Read the model definition and answer for the solid it produces. Units are mm, in the model's axes. Face numbers are marked on the shaded views. A direction names the side the tool comes from. Round coordinates to 2 decimals unless told otherwise and drop trailing zeros. Write each loop counter-clockwise with the first axis right and the second up, starting at its lowest first coordinate (ties: lowest second). Pieces come first, ordered by that corner, then holes. Notation, with made-up numbers: (61.5, 86) - (114.5, 86) arc R25 cw to (114.5, 119) - close; hole circle Ø8 at (73.5, -33.5). An arc over 180 degrees is marked (long way). Answer as CSV lines item,"result". Start each with the question number.
1) Which of the six approach directions +Z, -Z, +X, -X, +Y, -Y give full straight-line access (tool end or side, diameter ignored) to the marked faces 5 and 6?
2) Find section D-D on x = 16.5. Determine the outline of the cut face in (y, z), then the cut area to 3 significant figures.
3) Consider line 1 along Z through (x, y) = (-17, 6.5); line 2 along Y through (x, z) = (-32.5, 33.5); line 3 along Z through (x, y) = (-34, 47.5). Determine where each line is inside the solid, lowest interval first.
4) Find section B-B on x = 31. Determine the outline of the cut face in (y, z), then the cut area to 3 significant figures.
5) For a pull along X with two mould halves and no side action, classify the marked faces 1, 2, 3 and 4 as +X half, -X half, draft (parallel to the pull), parting line (faces both ways), or undercut.
6) Find section A-A on z = 4.5. Determine the outline of the cut face in (x, y), then the cut area to 3 significant figures.
7) Each of these flat-tipped pins is pushed along its axis until it touches: pin 1 (4.5 mm diameter, centred on x = -36, y = -2.5, fed in from -Z); pin 2 (1.2 mm diameter, centred on x = -14.5, z = 26, fed in from -Y); pin 3 (23 mm diameter, centred on x = 3.5, y = 30, fed in from +Z). Where does it stop, or does it pass through?
8) Find section C-C on y = -3. Determine the outline of the cut face in (x, z), then the cut area to 3 significant figures.
from build123d import *

# Parameters (mm, degrees)
F0_W      = 76.35137
F0_H      = 104.6798825264
F1_DEPTH  = 20
F3_DEPTH  = 105
F4_W      = 93.6356825264
F4_H      = 10
F5_DEPTH  = 100
F7_DEPTH  = 25
F6_W      = 71.0693526958
F6_H      = 99.8780601819
F8_DEPTH  = 5
F9_W      = 29.2911557481
F9_H      = 16.3262225688
F9_W_2    = 29.291
F10_DEPTH = 4
F11_R     = 1.65


with BuildPart() as f1:
    # F0 (on Top) → F1 (new body)
    with BuildSketch(Plane.XY):
        with Locations((-0.238945, 18.4870436788)):
            Rectangle(F0_W, F0_H)
    extrude(amount=F1_DEPTH)

    # F2 (on face) → F3 (cut)
    with BuildSketch(Plane.XZ.offset(33.8528975844)):
        Polygon((32.4146378825, 10.8041167259), (-32.89253, 10.8041167259), (-32.89253, 9.3744061509), (-32.89253, 0), (32.4146378825, 0), (32.4146378825, 9.3744061509), align=None)
    extrude(amount=-F3_DEPTH, mode=Mode.SUBTRACT)

    # F4 (on face) → F5 (cut)
    with BuildSketch(Plane(origin=(-38.41463, 0, 0), x_dir=(0, -1, 0), z_dir=(-1, 0, 0))):
        with Locations((-18.4870436788, 5)):
            Rectangle(F4_W, F4_H)
    extrude(amount=-F5_DEPTH, mode=Mode.SUBTRACT)

    # F6 (on face) → F7 (join)
    with BuildSketch(Plane.XY.offset(20)):
        Polygon((-38.41463, 68.4260725975), (-35.7736226958, 68.4260725975), (35.29573, 68.4260725975), (37.93674, 68.4260725975), (37.93674, 70.826984942), (-38.41463, 70.826984942), align=None)
    extrude(amount=F7_DEPTH)

    # F6 (on face) → F8 (join)
    with BuildSketch(Plane.XY.offset(20)):
        with Locations((-0.2389463479, 18.4870425065)):
            Rectangle(F6_W, F6_H)
    extrude(amount=F8_DEPTH)

    # F9 (on face) → F10 (join)
    with BuildSketch(Plane.XY.offset(25)):
        with Locations((-17.5266725798, 57.14177154)):
            Rectangle(F9_W, F9_H)
        with Locations((14.4065536521, 57.14177154)):
            Rectangle(F9_W_2, F9_H)
    extrude(amount=F10_DEPTH)

    # F11
    f11_edges = [f1.edges().sort_by_distance(p)[0] for p in [
        (-17.526673, 48.97866, 29),
        (-32.17225, 65.304883, 27),
        (-0.238946, 48.97866, 27),
        (14.406554, 48.97866, 29),
        (-0.238946, 57.141772, 29),
        (-32.17225, 57.141772, 29),
        (-32.17225, 48.97866, 27),
        (-2.881095, 48.97866, 27),
        (-2.881095, 57.141772, 29),
        (29.052054, 57.141772, 29),
        (29.052054, 48.97866, 27),
    ]]
    fillet(f11_edges, radius=F11_R)


solid = f1.part
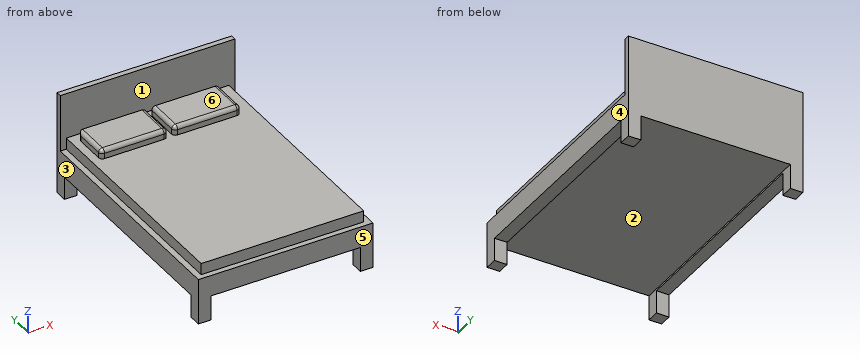
Check values:
1,face 5,"+Z, -Z, +X, -X, -Y"
1,face 6,"+Z, +X, -X, -Y"
2,outline,"(-33.85, 10.8) - (70.83, 10.8) - (70.83, 45) - (68.43, 45) - (68.43, 25) - (65.3, 25) - (65.3, 29) - (50.63, 29) arc R1.65 ccw to (48.98, 27.35) - (48.98, 25) - (-31.45, 25) - (-31.45, 20) - (-33.85, 20) - close"
2,area,"1,590 mm^2"
3,line 1,"z = 10.8 to 25"
3,line 2,"y = 68.43 to 70.83"
3,line 3,"z = 10 to 25"
4,outline,"(-33.85, 10.8) - (70.83, 10.8) - (70.83, 45) - (68.43, 45) - (68.43, 25) - (-31.45, 25) - (-31.45, 20) - (-33.85, 20) - close"
4,area,"1,520 mm^2"
5,face 1,"draft"
5,face 2,"undercut"
5,face 3,"-X half"
5,face 4,"+X half"
6,outline,"(-38.41, -33.85) - (-32.89, -33.85) - (-32.89, -28.33) - (-38.41, -28.33) - close; (-38.41, 65.3) - (-32.89, 65.3) - (-32.89, 70.83) - (-38.41, 70.83) - close; (32.41, -33.85) - (37.94, -33.85) - (37.94, -28.33) - (32.41, -28.33) - close; (32.41, 65.3) - (37.94, 65.3) - (37.94, 70.83) - (32.41, 70.83) - close"
6,area,"122 mm^2"
7,pin 1,"stops at z = 10"
7,pin 2,"stops at y = 48.98"
7,pin 3,"stops at z = 25"
8,outline,"(-38.41, 10) - (-32.89, 10) - (-32.89, 10.8) - (32.41, 10.8) - (32.41, 10) - (37.94, 10) - (37.94, 20) - (35.3, 20) - (35.3, 25) - (-35.77, 25) - (-35.77, 20) - (-38.41, 20) - close"
8,area,"1,070 mm^2"
